Autodesk Inventor part; units mm, degrees
ref_plane "YZ Plane" through (0, 0, 0) normal (1, 0, 0) x (0, 1, 0)
ref_plane "XZ Plane" through (0, 0, 0) normal (0, 1, 0) x (-1, 0, 0)
ref_plane "XY Plane" through (0, 0, 0) normal (0, 0, 1) x (1, 0, 0)
sketch "Sketch1" plane through (0, 0, 0) normal (0, 0, 1) x (1, 0, 0)
  circle A0 centre (0, 0) radius 7.5
  line L0 (0, 7.5) -> (-2.5, 7.5)
  line L1 (-2.5, 7.5) -> (-2.5, 4.5)
  line L2 (-2.5, 4.5) -> (0, 4.5)
  line L3 (0, 4.5) -> (0, 7.5)
  line L4 (0, 7.5) -> (2.5, 7.5)
  line L5 (2.5, 7.5) -> (2.5, 4.5)
  line L6 (2.5, 4.5) -> (0, 4.5)
  point P0 (-2.5, 7.0711)
  point P1 (2.5, 7.0711)
  dimension "d0" = 15
  dimension "d1" = 3
  dimension "d2" = 2.5
extrude "Extrusion1" add sketch "Sketch1" along normal blind 110 contours A0 L1 L2 L6 L5
properties part number "shaft_with_keyway"
Design review of the part built by this model. Coordinates are the model's own, in mm. A direction names the side the tool comes from. Coordinates: 2 decimals unless noted, no trailing zeros. Write each loop counter-clockwise with the first axis right and the second up, starting at its lowest first coordinate (ties: lowest second). Pieces come first, ordered by that corner, then holes. Notation, with made-up numbers: M 70,35.25 L 105,35.25 A15 ccw 105,59.25 Z; hole C 5,-5.5 d5. An arc over 180 degrees is marked long. Answer as a JSON object with one key per item and string values.
Item 1: Draft analysis for pull direction X (two halves, no side actions). For faces 1 (the cylindrical face through (0.294, -7.494, 54.23)), 2 (the flat face through (2.5, 6, 54)), 3 (the flat face through (0, 0, 110)), state which applies: pulls with the +X half, pulls with the -X half, needs draft (parallel to the pull), parting line crosses it, or undercut.
Outcome:
{"face 1": "parting line crosses it", "face 2": "undercut", "face 3": "needs draft"}
Item 2: Add section A-A, the plane x = 6. Give the boundary of the cut face in (y, z).
Outcome:
{"outline": "M -4.5,0 L 4.5,0 L 4.5,110 L -4.5,110 Z"}
Item 3: Machinability: for faces 4 (the flat face through (0, 0, 0)), 5 (the flat face through (-2.5, 6, 54)), which of the approach directions +Z, -Z, +X, -X, +Y, -Y give a long, thin tool a straight path to every point of the face, cutting with its end or side? Answer none if there is none.
Outcome:
{"face 4": "-Z, +X, -X, +Y, -Y", "face 5": "+Z, -Z, +Y"}
Item 4: Insertion check: pin 1 Ø1 at (y, z) = (-1, 81) entering from -X; pin 2 Ø1.3 at (y, z) = (5.5, 63) entering from -X; pin 3 Ø3 at (x, z) = (3.5, 25.5) entering from -Y. Each pin has a flat end and moves straight along its axis. Give the tip position at first contact, or say it passes through.
Outcome:
{"pin 1": "x = -7.48", "pin 2": "x = -5.72", "pin 3": "y = -7.23"}
Item 5: Add section B-B, the plane z = 95. Give the boundary of the cut face in (x, y), and give its area (3 significant figures).
Outcome:
{"outline": "M -2.5,4.5 L -2.5,7.07 A7.5 ccw long 2.5,7.07 L 2.5,4.5 Z", "area": "162 mm²"}
Item 6: Wall thickness on probe 1 along Y at (x, z) = (2.75, 34.5); probe 2 along Y at (x, z) = (-2, 19.5); probe 3 along X at (y, z) = (0.5, 8.5): over which ranges is each line inside the solid? List them lowest first.
Outcome:
{"probe 1": "-6.98 to 6.98", "probe 2": "-7.23 to 4.5", "probe 3": "-7.48 to 7.48"}
